from build123d import *

# Parameters (mm, degrees)
BOSS_EXTRUDE1_DEPTH      = 5
BOSS_EXTRUDE1_DEPTH_BACK = 5


with BuildPart() as part:
    # Sketch1 → Boss-Extrude1 (new body, two sides)
    with BuildSketch(Plane.XY) as boss_extrude1_sk:
        Polygon((-4.3, 2.9), (-4.3, -2.9), (-0.8, -5), (-0.8, -2.9), (0, -2.9), (0, 2.9), (-0.8, 2.9), (-0.8, 5), align=None)
    extrude(amount=BOSS_EXTRUDE1_DEPTH)
    extrude(boss_extrude1_sk.sketch, amount=-BOSS_EXTRUDE1_DEPTH_BACK)

    # Sketch2 → Cut-Revolve1 (revolve, cut)
    with BuildSketch(Plane.XY):
        Polygon((-4.3, 0), (-4.3, 2.5), (-3.867, 2.067), (-0.433, 2.067), (0, 2.5), (0, 0), align=None)
    revolve(axis=Axis((0, 0, 0), (-1, 0, 0)), mode=Mode.SUBTRACT)


solid = part.part
Here's how the part is built. I have some questions about the finished solid (model axes, mm). A direction names the side the tool comes from. Coordinates: 2 decimals unless noted, no trailing zeros. Order: outer loops, then holes, each group sorted by start corner. A loop starts at its lowest first (then second) coordinate and runs counter-clockwise, first axis right, second up. Notation, with made-up numbers: M 15,-20 L 68,-20 A20 cw 68,-4 Z; hole C 54,11.5 d10. An arc over 180 degrees is marked long. Answer as CSV lines item,"result". Start each with the question number.
1. I want a section at C-C, the plane z = 0. Write out the boundary of the cut face in (x, y).
2. I want a section at B-B, the plane x = -2.6. Write out the boundary of the cut face in (y, z).
3. I want a section at A-A, the plane y = 0. Write out the boundary of the cut face in (x, z).
4. I want a section at D-D, the plane z = 2.75. Write out the boundary of the cut face in (x, y).
5. I need wall thicknesses on line 1 (Z direction, x = -2.4, y = 0); line 2 (Y direction, x = -3.7, z = 0.5); line 3 (Z direction, x = -2.4, y = 0.75). Which ranges of each line are inside material? Lowest first, please. Write a range as [from, to].
6. We'd pull the mould along Z, two halves only. Please class faces 1 (the flat face through (-2, 0, -5)), 2 (the cylindrical face through (-2.13, -1.64, 1.26)), 3 (the flat face through (-2, 0, 5)), 4 (the flat face through (-0.8, 4, 0)): released by +Z, released by -Z, zero draft, split by the parting line, or undercut.
7. For pin 1 (2 mm diameter, centred on x = -3, z = -3.5, fed in from +Y); pin 2 (1 mm diameter, centred on y = 4, z = -1.5, fed in from +X); pin 3 (0.6 mm diameter, centred on x = 0, z = -1, fed in from -Y); pin 4 (3.5 mm diameter, centred on y = 0, z = 0, fed in from -X), each with a flat end and sliding along its axis, tell me the tip position at first contact or that it passes through.
8. On a 3-axis mill with a long thin cutter (end or side, diameter ignored), from which of +Z, -Z, +X, -X, +Y, -Y can I reach the whole of each face in a straight line? I mean faces 5 (the flat face through (-0.8, -4, 0)), 6 (the flat face through (-2.57, -3.94, 0.07)). Say none if no direction works.
Recorded:
1,outline,"M -4.3,-2.9 L -0.8,-5 L -0.8,-2.9 L 0,-2.9 L 0,-2.5 L -0.43,-2.07 L -3.87,-2.07 L -4.3,-2.5 Z; M -4.3,2.5 L -3.87,2.07 L -0.43,2.07 L 0,2.5 L 0,2.9 L -0.8,2.9 L -0.8,5 L -4.3,2.9 Z"
2,outline,"M -3.92,-5 L 3.92,-5 L 3.92,5 L -3.92,5 Z; hole C 0,0 d4.13"
3,outline,"M -4.3,-5 L 0,-5 L 0,-2.5 L -0.43,-2.07 L -3.87,-2.07 L -4.3,-2.5 Z; M -4.3,2.5 L -3.87,2.07 L -0.43,2.07 L 0,2.5 L 0,5 L -4.3,5 Z"
4,outline,"M -4.3,-2.9 L -0.8,-5 L -0.8,-2.9 L 0,-2.9 L 0,2.9 L -0.8,2.9 L -0.8,5 L -4.3,2.9 Z"
5,line 1,"z = [-5, -2.07], [2.07, 5]"
5,line 2,"y = [-3.26, -2.01], [2.01, 3.26]"
5,line 3,"z = [-5, -1.93], [1.93, 5]"
6,face 1,"released by -Z"
6,face 2,"undercut"
6,face 3,"released by +Z"
6,face 4,"zero draft"
7,pin 1,"stops at y = 4.28"
7,pin 2,"stops at x = -0.8"
7,pin 3,"stops at y = -2.9"
7,pin 4,"passes through"
8,face 5,"+Z, -Z, +X, -Y"
8,face 6,"+Z, -Z, -X, -Y"
